Source: three-view drawing plus pictorial views. Frame: mm from the lowest corner of the part. A direction names the side the tool comes from. Give positions to 0.01 mm unless a question says otherwise; leave off trailing zeros. Order: outer loops, then holes, each group sorted by start corner. A loop starts at its lowest first (then second) coordinate and runs counter-clockwise, first axis right, second up.
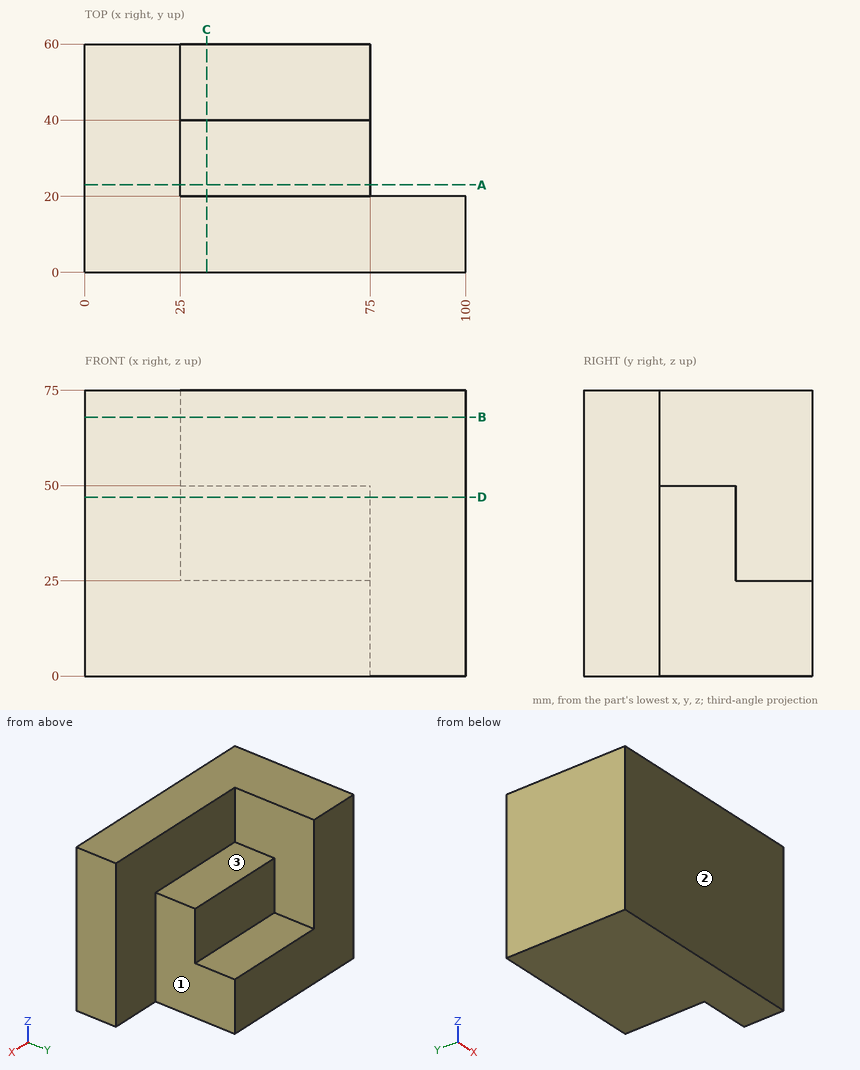
(1) Section A-A, the plane y = 23. Return loops of the section in (x, z), plus the area to 4 significant figures.
(2) Section B-B, the plane z = 68. Return loops of the section in (x, y), plus the area to 3 significant figures.
(3) Line query: line 1 along Y through (x, z) = (93.5, 57.5); line 2 along Y through (x, z) = (54, 28); line 3 along Z through (x, y) = (29.5, 51). Output: solid intervals per line, ascending.
(4) Section D-D, the plane z = 47. Return loops of the section in (x, y).
(5) Access query for the marked faces 1, 2 and 3. Directions: +Z, -Z, +X, -X, +Y, -Y. A direction counts if a zero-diameter tool reaches every point of the face in a straight line with its end or side. Return the directions, or none.
(6) Section C-C, the plane x = 32. Return loops of the section in (y, z), plus the area to 3 significant figures.
(7) Pin query (flat end, axial travel): pin 1 Ø12 at (y, z) = (42, 62) entering from +X; pin 2 Ø1 at (x, y) = (35, 34.5) entering from +Z; pin 3 Ø5 at (x, z) = (82, 21.5) entering from +Y. Return the tip coordinate at first contact, or that it passes through.
Checks:
1. outline: (0, 0) - (75, 0) - (75, 50) - (25, 50) - (25, 75) - (0, 75) - close
1. area: 4,375 mm2
2. outline: (0, 0) - (100, 0) - (100, 20) - (25, 20) - (25, 60) - (0, 60) - close
2. area: 3,000 mm2
3. line 1: y = 0 to 20
3. line 2: y = 0 to 40
3. line 3: z = 0 to 25
4. outline: (0, 0) - (100, 0) - (100, 20) - (75, 20) - (75, 40) - (25, 40) - (25, 60) - (0, 60) - close
5. face 1: +Z, -Z, +X, +Y
5. face 2: +Z, -Z, +X, -X, -Y
5. face 3: +Z, +X, +Y
6. outline: (0, 0) - (60, 0) - (60, 25) - (40, 25) - (40, 50) - (20, 50) - (20, 75) - (0, 75) - close
6. area: 3,000 mm2
7. pin 1: stops at x = 25
7. pin 2: stops at z = 50
7. pin 3: stops at y = 20
